Autodesk Inventor part; units mm, degrees
ref_plane "YZ Plane" through (0, 0, 0) normal (1, 0, 0) x (0, 1, 0)
ref_plane "XZ Plane" through (0, 0, 0) normal (0, 1, 0) x (-1, 0, 0)
ref_plane "XY Plane" through (0, 0, 0) normal (0, 0, 1) x (1, 0, 0)
sketch "Эскиз3" plane through (0, 0, 0) normal (0, 0, 1) x (1, 0, 0)
  line L0 (110.155, -68.7957) -> (60.155, -68.7957) construction
  line L1 (60.155, -68.7957) -> (60.155, 68.0464) construction
  line L2 (110.155, 68.0464) -> (110.155, -68.7957) construction
  circle A0 centre (57.105, -53.7957) radius 3.05
  circle A1 centre (57.105, -13.7957) radius 3.05
  circle A2 centre (57.105, 26.2043) radius 3.05
  circle A3 centre (113.205, -53.7957) radius 3.05
  circle A4 centre (113.205, -13.7957) radius 3.05
  circle A5 centre (113.205, 26.2043) radius 3.05
  circle A6 centre (85.155, -78.7957) radius 10
  line L3 (85.155, -21.4404) -> (85.155, -113.936) construction
  arc A7 (119.305, 26.2043) -> (113.205, 32.3043) centre (113.205, 26.2043) ccw
  arc A8 (57.105, 32.3043) -> (51.005, 26.2043) centre (57.105, 26.2043) ccw
  line L4 (113.205, 32.3043) -> (57.105, 32.3043)
  line L5 (119.305, 26.2043) -> (119.305, -78.7957)
  line L6 (51.005, 26.2043) -> (51.005, -78.7957)
  arc A9 (51.005, -78.7957) -> (119.305, -78.7957) centre (85.155, -78.7957) ccw
  circle A10 centre (66.205, -33.7957) radius 3.05
  circle A11 centre (66.205, 6.2043) radius 3.05
  circle A12 centre (104.105, -33.7957) radius 3.05
  circle A13 centre (104.105, 6.2043) radius 3.05
  point P0 (0, 0)
  dimension "d8" = 50
  dimension "d11" = 40
  dimension "d14" = 56.1
  dimension "d17" = 6.1
  dimension "d18" = 15
  dimension "d19" = 20
  dimension "d20" = 12.2
  dimension "d21" = 12.2
  dimension "d24" = 40
  dimension "d27" = 37.9
  dimension "d30" = 20
extrude "Выдавливание3" add sketch "Эскиз3" along normal blind 3
equation "\"d8\" = hight_profile_femur"
equation "\"d14\" = hight_profile_femur + d_main_screw_holes"
equation "\"d17\" = d_main_screw_holes"
equation "\"d19\" = d_main_shaft"
equation "\"d20\" = 2 * d_main_screw_holes"
equation "\"d21\" = 2 * d_main_screw_holes"
equation "\"d27\" = -d_main_screw_holes + hight_profile_femur - 2 * thickness_profile_femur"
equation "\"d6\" = thickness_steel"
equation "\"tolerance_plazma\" = 0.1"
equation "\"thickness_steel\" = 3"
equation "\"d_main_screw_holes\" = 6.1"
equation "\"d_main_shaft\" = 20"
equation "\"thickness_profile_tibea\" = 4"
equation "\"thickness_profile_femur\" = 3"
equation "\"width_shaft_shift\" = 35"
equation "\"hight_profile_femur\" = 50"
equation "\"width_flattened_surface\" = 12"
properties part number "femur_outside_steel" material "Сталь"
Can you work these out from the model? Positions are in its coordinate system, mm. Give positions to 0.01 mm unless a question says otherwise; leave off trailing zeros. Loops run counter-clockwise (first coordinate to the right, second up) from the corner with the lowest first, then second, coordinate; pieces in that order, holes last. Notation, with made-up numbers: (-34, 15) - (0, 15) arc R14 cw to (0, 23) - close; hole circle Ø10 at (-17.5, -37). An arc over 180 degrees is marked (long way). One line per item, written item: value.
(1) I'm going to push flat-ended pins straight in: pin 1 (10 mm diameter, centred on x = 113.2, y = -13.8, fed in from +Z); pin 2 (16 mm diameter, centred on x = 85.16, y = -78.8, fed in from +Z); pin 3 (1.5 mm diameter, centred on x = 110, z = 2.5, fed in from -Y). Where does each tip first touch, or does it pass through?
Verdict:
pin 1: z = 3
pin 2: through
pin 3: y = -103
(2) If we section it at C-C, the plane x = 91: List the corners of the cut face in (y, z) for me.
Verdict:
outline: (-112.44, 0) - (-86.91, 0) - (-86.91, 3) - (-112.44, 3) - close; (-70.68, 0) - (32.3, 0) - (32.3, 3) - (-70.68, 3) - close
(3) If we section it at A-A, the plane x = 103: List the corners of the cut face in (y, z) for me.
Verdict:
outline: (-107.91, 0) - (-36.64, 0) - (-36.64, 3) - (-107.91, 3) - close; (-30.95, 0) - (3.36, 0) - (3.36, 3) - (-30.95, 3) - close; (9.05, 0) - (32.3, 0) - (32.3, 3) - (9.05, 3) - close
(4) If we section it at D-D, the plane z = 1.95: State how many separate pieces and enclosed holes the cut face has, plus the area to 3 significant figures.
Verdict:
separate pieces: 1
enclosed holes: 11
area: 8,800 mm^2
(5) If we section it at B-B, the plane y = -32.5: List the corners of the cut face in (x, z) for me (3 decimals).
Verdict:
outline: (51.005, 0) - (63.444, 0) - (63.444, 3) - (51.005, 3) - close; (68.966, 0) - (101.344, 0) - (101.344, 3) - (68.966, 3) - close; (106.866, 0) - (119.305, 0) - (119.305, 3) - (106.866, 3) - close
(6) I need wall thicknesses on line 1 along Y through (x, z) = (65.5, 2.8); line 2 along X through (y, z) = (25, 0.4) (3 decimals); line 3 along X through (y, z) = (-52, 0.9) (3 decimals). Which ranges of each line are inside material? Lowest first, please.
Verdict:
line 1: -106.72 to -36.76, -30.83 to 3.24, 9.17 to 32.3
line 2: 51.005 to 54.303, 59.907 to 110.403, 116.007 to 119.305
line 3: 51.005 to 54.64, 59.57 to 110.74, 115.67 to 119.305
(7) If we mould it in two halves opening along X, with no side actions, what happens to faces 1 (the face through (110.158, -53.93, 1.479)), 2 (the face through (119.305, -26, 1)), 3 (the face through (85, -39, 0))? For each: released by +X, released by -X, zero draft, split by the parting line, or undercut.
Verdict:
face 1: undercut
face 2: released by +X
face 3: zero draft
